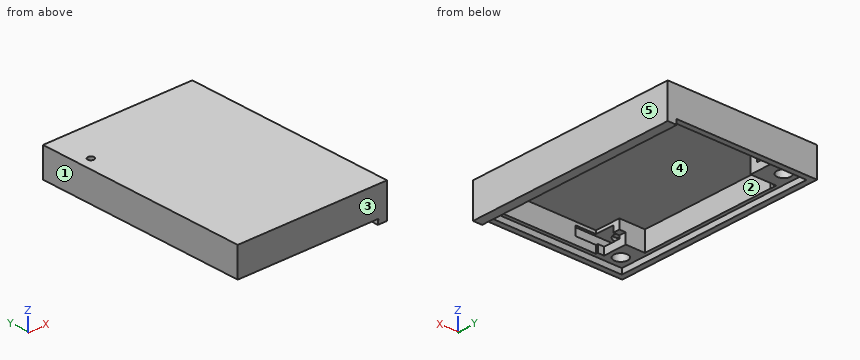
Solid Edge part; units mm, degrees
sketch "Sketch1" plane through (0, 0, 0) normal (0, 0, 1) x (1, 0, 0)
  line L0 (45.72, -2.54) -> (45.72, 66.04)
  line L1 (45.72, 66.04) -> (-2.54, 66.04)
  line L2 (-2.54, 66.04) -> (-2.54, -2.54)
  line L3 (-2.54, -2.54) -> (45.72, -2.54)
  line L4 (42.799, 0.381) -> (42.799, 63.119)
  line L5 (42.799, 63.119) -> (0.381, 63.119)
  line L6 (0.381, 63.119) -> (0.381, 0.381)
  line L7 (0.381, 0.381) -> (42.799, 0.381)
extrude "Protrusion1" add sketch "Sketch1" along normal blind 6.35
sketch "Sketch2" plane through (21.59, 31.75, 0) normal (0, 0, -1) x (0, 1, 0)
  line L0 (32.512, -22.352) -> (32.512, 22.352)
  line L1 (32.512, 22.352) -> (-32.512, 22.352)
  line L2 (-32.512, 22.352) -> (-32.512, -22.352)
  line L3 (-32.512, -22.352) -> (32.512, -22.352)
  line L4 (34.29, 24.13) -> (34.29, -24.13)
  line L5 (34.29, -24.13) -> (-34.29, -24.13)
  line L6 (-34.29, -24.13) -> (-34.29, 24.13)
  line L7 (-34.29, 24.13) -> (34.29, 24.13)
extrude "Protrusion2" add sketch "Sketch2" along normal up to vertex (1.778 mm away)
sketch "Sketch3" plane through (21.59, -2.54, 2.286) normal (0, -1, 0) x (-1, 0, 0)
  line L0 (-24.13, 5.6414) -> (-21.187, 5.6414)
  line L1 (-21.187, 5.6414) -> (-21.336, 4.064)
  line L2 (-21.336, 4.064) -> (-24.13, 4.064)
  line L3 (-24.13, 4.064) -> (-24.13, 5.6414)
extrude "Protrusion3" add sketch "Sketch3" against normal up to vertex (68.58 mm away)
sketch "Sketch4" plane through (21.59, 31.75, 6.35) normal (0, 0, 1) x (0, -1, 0)
  line L0 (34.29, 24.13) -> (-34.29, 24.13)
  line L1 (-34.29, 24.13) -> (-34.29, -24.13)
  line L2 (-34.29, -24.13) -> (34.29, -24.13)
  line L3 (34.29, -24.13) -> (34.29, 24.13)
extrude "ExtrudedProtrusion_4" add sketch "Sketch4" along normal blind 1.27
sketch "Sketch5" plane through (21.59, 31.75, 0) normal (0, 0, -1) x (-1, 0, 0)
  line L0 (12.95, -23.11) -> (24.13, -23.11)
  line L1 (24.13, -23.11) -> (24.13, -34.29)
  line L2 (24.13, -34.29) -> (12.95, -34.29)
  line L3 (12.95, -34.29) -> (12.95, -23.11)
  line L4 (12.95, 34.29) -> (12.95, 23.098)
  line L5 (12.95, 23.098) -> (24.13, 23.098)
  line L6 (24.13, 23.098) -> (24.13, 34.29)
  line L7 (24.13, 34.29) -> (12.95, 34.29)
extrude "Protrusion4" add sketch "Sketch5" against normal up to vertex (7.62 mm away)
sketch "Sketch6" plane through (21.59, 31.75, 0) normal (0, 0, -1) x (1, 0, 0)
  circle A0 centre (-18.54, -28.694) radius 2.2179
  circle A1 centre (-18.539, 28.7065) radius 2.2179
extrude "Cutout1" cut sketch "Sketch6" against normal up to vertex (6.35 mm away)
sketch "Sketch7" plane through (8.64, 4.0083, 3.175) normal (1, 0, 0) x (0, 0, 1)
  line L0 (2.1584, -2.4641) -> (-0.7626, -2.4641)
  line L1 (-0.7626, -2.4641) -> (-0.7626, 4.3939)
  line L2 (-0.7626, 4.3939) -> (2.1584, 4.3939)
  line L3 (2.1584, 4.3939) -> (2.1584, -2.4641)
  line L4 (-0.7626, -53.0066) -> (2.1584, -53.0066)
  line L5 (2.1584, -53.0066) -> (2.1584, -59.8646)
  line L6 (2.1584, -59.8646) -> (-0.7626, -59.8646)
  line L7 (-0.7626, -59.8646) -> (-0.7626, -53.0066)
extrude "ExtrudedCutout_2" cut sketch "Sketch7" along normal blind 6.604
sketch "Sketch8" plane through (8.64, 4.0083, 3.175) normal (1, 0, 0) x (0, 0, 1)
  line L0 (2.1584, -2.4641) -> (-0.7626, -2.4641)
  line L1 (-0.7626, -2.4641) -> (-0.7626, 4.3939)
  line L2 (-0.7626, 4.3939) -> (2.1584, 4.3939)
  line L3 (2.1584, 4.3939) -> (2.1584, -2.4641)
  line L4 (-0.7626, -59.8646) -> (-0.7626, -53.0066)
  line L5 (-0.7626, -53.0066) -> (2.1584, -53.0066)
  line L6 (2.1584, -53.0066) -> (2.1584, -59.8646)
  line L7 (2.1584, -59.8646) -> (-0.7626, -59.8646)
extrude "ExtrudedCutout_3" cut sketch "Sketch8" against normal blind 10.16
sketch "Sketch9" plane through (21.59, 31.75, 7.62) normal (0, 0, 1) x (0, 1, 0)
  circle A0 centre (21.58, 20.33) radius 1.016
extrude "Cutout2" cut sketch "Sketch9" against normal through all
sketch "Sketch10" plane through (21.59, 31.75, 0) normal (0, 0, -1) x (0, 1, 0)
  line L0 (-30.734, -14.9831) -> (-23.11, -14.9831)
  line L1 (-23.11, -14.9831) -> (-23.11, -12.95)
  line L2 (-23.11, -12.95) -> (-30.734, -12.95)
  line L3 (-30.734, -12.95) -> (-30.734, -14.9831)
extrude "ExtrudedCutout_6" cut sketch "Sketch10" against normal blind 3.34
Can you work these out from the model? Positions are in its coordinate system, mm. Face numbers are marked on the shaded views. A direction names the side the tool comes from. Round coordinates to 2 decimals unless told otherwise and drop trailing zeros. Loops run counter-clockwise (first coordinate to the right, second up) from the corner with the lowest first, then second, coordinate; pieces in that order, holes last. Notation, with made-up numbers: M 71.25,-7.5 L 127.25,-7.5 A26 ccw 127.25,29.5 Z; hole C 39.5,-31.5 d7. An arc over 180 degrees is marked long. Answer as a JSON object with one key per item and string values. Group by question number.
Q1. We'd pull the mould along Y, two halves only. Please class the marked faces 3, 4 and 5: +Y half, -Y half, draft (parallel to the pull), parting line (faces both ways), or undercut.
Q2. Imagine slicing it at D-D, the plane x = 40. Please give me the cut outline in (y, z), then the cut area to 3 significant figures.
Q3. Please list where these lines run through material, in increasing order: L1, parallel to Y at x = 3.05, z = 5.75; L2, parallel to X at y = 30.5, z = 5.75; L3, parallel to Y at x = 29.5, z = 1.25.
Q4. Imagine slicing it at B-B, the plane x = 12. Please give me the cut outline in (y, z), then the cut area to 3 significant figures.
Q5. Imagine slicing it at A-A, the plane z = -1. Please give me the cut outline in (x, y).
Q6. On a 3-axis mill with a long thin cutter (end or side, diameter ignored), from which of +Z, -Z, +X, -X, +Y, -Y can I reach the whole of each face in a straight line? I mean the marked faces 1 and 2. Say none if no direction works.
Q7. Imagine slicing it at C-C, the plane y = 25. Please give me the cut outline in (x, z).
Q8. Will these pins go through, and if not, where does the flat tip stop? pin 1 (1.3 mm diameter, centred on x = 2, y = 60.5, fed in from -Z); pin 2 (3.5 mm diameter, centred on x = 3, y = 2, fed in from -Z).
Findings:
{
 "1": {"face 3": "-Y half", "face 4": "undercut", "face 5": "draft"},
 "2": {"outline": "M -2.54,-1.78 L -0.76,-1.78 L -0.76,0 L 0.38,0 L 0.38,6.35 L 63.12,6.35 L 63.12,0 L 64.26,0 L 64.26,-1.78 L 66.04,-1.78 L 66.04,7.62 L -2.54,7.62 Z", "area": "131 mm2"},
 "3": {"L1": "y = -2.54 to 0.83, 5.26 to 8.64, 54.85 to 58.23, 62.66 to 66.04", "L2": "x = -2.54 to 0.38, 42.8 to 45.72", "L3": "y = -2.54 to 0.38, 63.12 to 66.04"},
 "4": {"outline": "M -2.54,-1.78 L -0.76,-1.78 L -0.76,0 L 0.38,0 L 0.38,2.41 L -0.39,2.41 L -0.39,5.33 L 0.38,5.33 L 0.38,6.35 L 63.12,6.35 L 63.12,5.33 L 63.87,5.33 L 63.87,2.41 L 63.12,2.41 L 63.12,0 L 64.26,0 L 64.26,-1.78 L 66.04,-1.78 L 66.04,7.62 L -2.54,7.62 Z", "area": "126 mm2"},
 "5": {"outline": "M -2.54,-2.54 L 45.72,-2.54 L 45.72,66.04 L -2.54,66.04 Z; hole M -0.76,-0.76 L 43.94,-0.76 L 43.94,64.26 L -0.76,64.26 Z"},
 "6": {"face 1": "+Z, -Z, -X, +Y, -Y", "face 2": "-Z"},
 "7": {"outline": "M -2.54,-1.78 L -0.76,-1.78 L -0.76,0 L 0.38,0 L 0.38,6.35 L 42.8,6.35 L 42.8,0 L 43.94,0 L 43.94,-1.78 L 42.93,-1.78 L 42.78,-3.36 L 45.72,-3.36 L 45.72,7.62 L -2.54,7.62 Z"},
 "8": {"pin 1": "stops at z = 6.35", "pin 2": "stops at z = 0"}
}
